```python
from build123d import *

# Parameters (mm, degrees)
CROQUIS1_R              = 45
SALIENTE_EXTRUIR1_DEPTH = 7
CROQUIS2_R              = 26.1
CORTAR_EXTRUIR1_DEPTH   = 8
CROQUIS3_R              = 4
CORTAR_EXTRUIR2_DEPTH   = 8


with BuildPart() as part:
    # Croquis1 → Saliente-Extruir1 (new body)
    with BuildSketch(Plane.XY):
        Circle(CROQUIS1_R)
    extrude(amount=SALIENTE_EXTRUIR1_DEPTH)

    # Croquis2 → Cortar-Extruir1 (cut, through all)
    with BuildSketch(Plane.XY.offset(7)):
        Circle(CROQUIS2_R)
    extrude(amount=-CORTAR_EXTRUIR1_DEPTH, mode=Mode.SUBTRACT)

    # Croquis3 → Cortar-Extruir2 (cut, through all)
    with BuildSketch(Plane.XY.offset(7)):
        with Locations((0, 35)):
            Circle(CROQUIS3_R)
        with Locations((35, 0)):
            Circle(CROQUIS3_R)
        with Locations((0, -35)):
            Circle(CROQUIS3_R)
        with Locations((-35, 0)):
            Circle(CROQUIS3_R)
    extrude(amount=-CORTAR_EXTRUIR2_DEPTH, mode=Mode.SUBTRACT)


solid = part.part
```
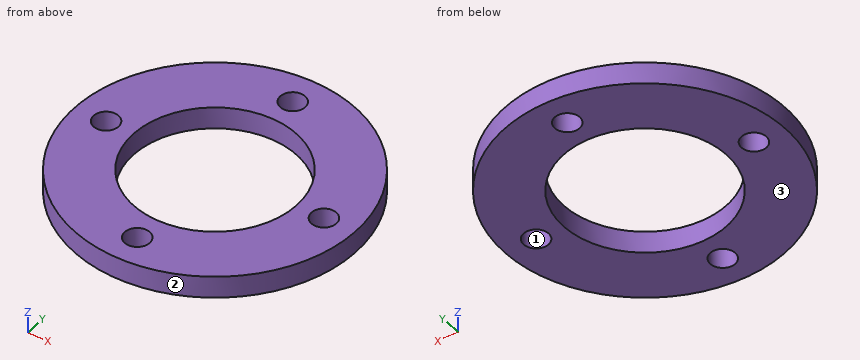
Read the model definition and answer for the solid it produces. Units are mm, in the model's axes. Face numbers are marked on the shaded views. Coordinates: 2 decimals unless noted, no trailing zeros. Write each loop counter-clockwise with the first axis right and the second up, starting at its lowest first coordinate (ties: lowest second). Pieces come first, ordered by that corner, then holes. Notation, with made-up numbers: (6.25, 18.25) -> (46.25, 18.25) arc R34 ccw to (46.25, 56.25) -> close; hole circle Ø5 at (2.25, 59). An arc over 180 degrees is marked (long way). Return JSON: item names as keys, results as strings.
1. A cutting plane is placed at C-C (x = -36.5). Determine the outline of the cut face in (y, z), and give its area (3 significant figures).
Found:
{"outline": "(-26.32, 0) -> (-3.71, 0) -> (-3.71, 7) -> (-26.32, 7) -> close; (3.71, 0) -> (26.32, 0) -> (26.32, 7) -> (3.71, 7) -> close", "area": "317 mm2"}
2. A cutting plane is placed at B-B (y = 35). Determine the outline of the cut face in (x, z).
Found:
{"outline": "(-28.28, 0) -> (-4, 0) -> (-4, 7) -> (-28.28, 7) -> close; (4, 0) -> (28.28, 0) -> (28.28, 7) -> (4, 7) -> close"}
3. Determine the mould class of the marked faces 1, 2 and 3 for opening direction Y: pulls with the +Y half, pulls with the -Y half, needs draft (parallel to the pull), parting line crosses it, or undercut.
Found:
{"face 1": "undercut", "face 2": "parting line crosses it", "face 3": "needs draft"}
4. A cutting plane is placed at A-A (x = 0). Determine the outline of the cut face in (y, z), and give its area (3 significant figures).
Found:
{"outline": "(-45, 0) -> (-39, 0) -> (-39, 7) -> (-45, 7) -> close; (-31, 0) -> (-26.1, 0) -> (-26.1, 7) -> (-31, 7) -> close; (26.1, 0) -> (31, 0) -> (31, 7) -> (26.1, 7) -> close; (39, 0) -> (45, 0) -> (45, 7) -> (39, 7) -> close", "area": "153 mm2"}
5. Each of these flat-tipped pins is pushed along its axis until it touches: P1, Ø1.5, axis at y = 2, z = 6, coming from the -X side; P2, Ø4, axis at y = -7.5, z = 2, coming from the -X side; P3, Ø1.5, axis at y = 32.5, z = 1.5, coming from the +X side. Where does it stop, or does it pass through?
Found:
{"P1": "x = -44.98", "P2": "x = -44.66", "P3": "x = 31.89"}
6. Find the intervals of material crossed by line 1 along Y through (x, z) = (0, 5); line 2 along Y through (x, z) = (-1.5, 1.75) (3 decimals); line 3 along X through (y, z) = (18, 2.25), in increasing order. Write a range as from..to.
Found:
{"line 1": "-45..-39, -31..-26.1, 26.1..31, 39..45", "line 2": "-44.975..-38.708, -31.292..-26.057, 26.057..31.292, 38.708..44.975", "line 3": "-41.24..-18.9, 18.9..41.24"}
7. A cutting plane is placed at D-D (z = 5.5). Determine the outline of the cut face in (x, y), and give its area (3 significant figures).
Found:
{"outline": "circle Ø90 at (0, 0); hole circle Ø8 at (-35, 0); hole circle Ø52.2 at (0, 0); hole circle Ø8 at (0, -35); hole circle Ø8 at (0, 35); hole circle Ø8 at (35, 0)", "area": "4,020 mm2"}
